Input: part model. Units: mm. Frame: model coordinates. A direction names the side the tool comes from. Give positions to 0.01 mm unless a question says otherwise; leave off trailing zeros. Loops run counter-clockwise (first coordinate to the right, second up) from the corner with the lowest first, then second, coordinate; pieces in that order, holes last. Notation, with made-up numbers: (-26, 68) -> (-9, 68) arc R35 ccw to (-9, 104) -> close; hole circle Ø5 at (-32, 21). An arc over 180 degrees is marked (long way). Answer in a Markdown table with one row per item. Add a question column.
```python
from build123d import *

# Parameters (mm, degrees)
FILLET1_R     = 3.175
CHAMFER1_SIZE = 3.175


with BuildPart() as part:
    # Sketch1 → Revolve1 (revolve)
    with BuildSketch(Plane.XY):
        Polygon((-6.35, 9.525), (-1.5875, 9.525), (-1.5875, -9.525), (-6.35, -9.525), (-6.35, -1.5875), (-28.575, -1.5875), (-28.575, -5.55625), (-33.3375, -5.55625), (-33.3375, 5.55625), (-28.575, 5.55625), (-28.575, 1.5875), (-6.35, 1.5875), align=None)
    revolve(axis=Axis((0, -9.525, 0), (0, 1, 0)))

    # Fillet1
    fillet1_edges = [part.edges().sort_by_distance(p)[0] for p in [
        (28.575, -1.5875, 0),
        (6.35, -1.5875, 0),
        (6.35, 1.5875, 0),
        (28.575, 1.5875, 0),
    ]]
    fillet(fillet1_edges, radius=FILLET1_R)

    # Chamfer1
    chamfer1_edges = [part.edges().sort_by_distance(p)[0] for p in [
        (33.3375, 5.55625, 0),
        (33.3375, -5.55625, 0),
    ]]
    chamfer(chamfer1_edges, length=CHAMFER1_SIZE)


solid = part.part
```
1) Section B-B on y = 0. Output: boundary loops of the cut face in (x, z) (1 decimal).
2) Section C-C on y = -3.75. Output: boundary loops of the cut face in (x, z) (1 decimal), and give its area (3 significant figures).
3) Material intervals for line 1 along Z through (x, y) = (0, -4.5); line 2 along X through (y, z) = (-4.75, 13); line 3 along Z through (x, y) = (0, 3), sorted ascending.
4) Section A-A on y = 3.5. Output: boundary loops of the cut face in (x, z) (1 decimal).
5) Pin query (flat end, axial travel): pin 1 (12 mm diameter, centred on x = -11.5, z = -25, fed in from +Y); pin 2 (1.5 mm diameter, centred on x = -24, z = -8.5, fed in from -Y); pin 3 (4 mm diameter, centred on y = 5.5, z = 9, fed in from +X); pin 4 (8 mm diameter, centred on y = 5, z = 0, fed in from -X). Return the tip coordinate at first contact, or that it passes through.
6) Reachability of faces 1 (the face through (1.3, -9.525, -1.3)), 2 (the face through (1.38, -7.11, -6.2)), 3 (the face through (28.547, 5.154, 1.256)) from +Z, -Z, +X, -X, +Y, -Y: full face, straight path, thin tool, end or side. Return the list, or none.
7) Pull-direction query (X, two-part tool) for faces 4 (the face through (24.094, -5.358, -18.474)), 5 (the face through (0.34, -0.13, -1.55)), 6 (the face through (-27, 5.556, -11)); classes: +X half, -X half, draft (parallel to the pull), parting line (faces both ways), or undercut.
Working result:
| question | item | result |
|---|---|---|
| 1 | outline | circle Ø66.7 at (0, 0); hole circle Ø3.2 at (0, 0) |
| 2 | outline | circle Ø63.9 at (0, 0); circle Ø13 at (0, 0); hole circle Ø56.8 at (0, 0); hole circle Ø3.2 at (0, 0) |
| 2 | area | 801 mm2 |
| 3 | line 1 | z = -31.22 to -28.56, -6.36 to -1.59, 1.59 to 6.36, 28.56 to 31.22 |
| 3 | line 2 | x = -28.11 to -25.45, 25.45 to 28.11 |
| 3 | line 3 | z = -32.72 to -28.04, -6.88 to -1.59, 1.59 to 6.88, 28.04 to 32.72 |
| 4 | outline | circle Ø64.4 at (0, 0); circle Ø13.2 at (0, 0); hole circle Ø56.6 at (0, 0); hole circle Ø3.2 at (0, 0) |
| 5 | pin 1 | stops at y = 5.56 |
| 5 | pin 2 | stops at y = -1.69 |
| 5 | pin 3 | stops at x = 31.01 |
| 5 | pin 4 | stops at x = -33.34 |
| 6 | face 1 | +Z, -Z, +X, -X, -Y |
| 6 | face 2 | -Y |
| 6 | face 3 | +Y |
| 7 | face 4 | parting line |
| 7 | face 5 | undercut |
| 7 | face 6 | draft |
